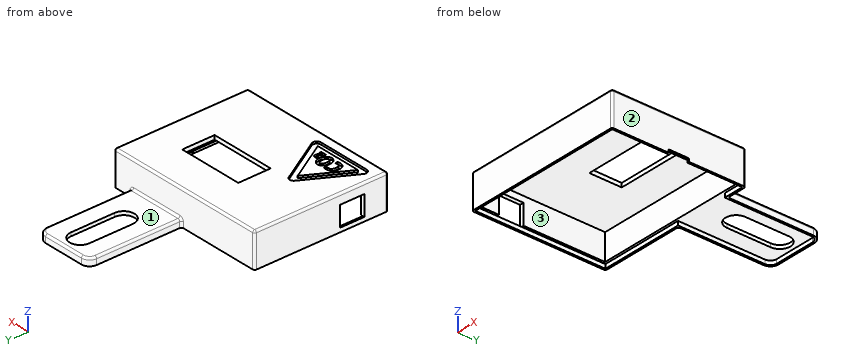
from build123d import *

# Parameters (mm, degrees)
CROQUIS1_W              = 80
CROQUIS1_H              = 66
SALIENTE_EXTRUIR2_DEPTH = 17
VACIADO7_T              = -2
CORTAR_EXTRUIR9_REACH   = 58.118
CROQUIS12_W             = 32
CROQUIS12_H             = 16
SALIENTE_EXTRUIR3_DEPTH = 3.75
CORTAR_EXTRUIR11_DEPTH  = 2
CORTAR_EXTRUIR26_REACH  = 117.461
CROQUIS16_W             = 10
CROQUIS16_H             = 12
CROQUIS20_RX            = 3.568577335
CROQUIS20_RY            = 2.914426882
CROQUIS20_RX_2          = 2.232634343
CROQUIS20_RY_2          = 1.215365865
CORTAR_EXTRUIR24_DEPTH  = 1
CORTAR_EXTRUIR25_REACH  = 117.461
CROQUIS27_W             = 1.5
CROQUIS27_H             = 10
REDONDEO3_R             = 1


with BuildPart() as part:
    # Croquis1 → Saliente-Extruir2 (new body)
    with BuildSketch(Plane.XY):
        with Locations((0, 2.5)):
            Rectangle(CROQUIS1_W, CROQUIS1_H)
    extrude(amount=SALIENTE_EXTRUIR2_DEPTH)

    # Vaciado7
    vaciado7_openings = [part.faces().sort_by_distance(p)[0] for p in [
        (0, 2.5, 0),
    ]]
    offset(amount=VACIADO7_T, openings=vaciado7_openings, kind=Kind.INTERSECTION)

    # Croquis12 → Cortar-Extruir9 (cut, up to next)
    with BuildSketch(Plane.XY.offset(17), mode=Mode.PRIVATE) as cortar_extruir9_sk1:
        with Locations((6.6, 9)):
            Rectangle(CROQUIS12_W, CROQUIS12_H)
    cortar_extruir9_tool1 = extrude(cortar_extruir9_sk1.sketch, amount=-CORTAR_EXTRUIR9_REACH, mode=Mode.PRIVATE) & part.part
    add(cortar_extruir9_tool1.solids().sort_by_distance((6.6, 9, 17))[0], mode=Mode.SUBTRACT)

    # Croquis29 → Saliente-Extruir3 (add)
    with BuildSketch(Plane(origin=(0, 0, 0), x_dir=(-1, 0, 0), z_dir=(0, 0, -1))):
        with BuildLine():
            Line((-1.5, 77.5), (-1.5, 35.5))
            Line((-1.5, 35.5), (-30, 35.5))
            Line((-30, 35.5), (-30, 77.5))
            ThreePointArc((-30, 77.5), (-28.828427125, 80.328427125), (-26, 81.5))
            Line((-26, 81.5), (-5.5, 81.5))
            ThreePointArc((-5.5, 81.5), (-2.671572875, 80.328427125), (-1.5, 77.5))
        make_face()
        with BuildLine():
            Line((-10.5, 73.25), (-10.5, 51.75))
            ThreePointArc((-10.5, 51.75), (-15.75, 46.5), (-21, 51.75))
            Line((-21, 51.75), (-21, 73.25))
            ThreePointArc((-21, 73.25), (-15.75, 78.5), (-10.5, 73.25))
        make_face(mode=Mode.SUBTRACT)
    extrude(amount=-SALIENTE_EXTRUIR3_DEPTH)

    # Croquis14 → Cortar-Extruir11 (cut)
    with BuildSketch(Plane(origin=(0, 0, 0), x_dir=(-1, 0, 0), z_dir=(0, 0, -1))):
        with BuildLine():
            Line((39.1, 34.6), (-2.4, 34.6))
            Line((-2.4, 34.6), (-2.4, 77.5))
            ThreePointArc((-2.4, 77.5), (-3.307968978, 79.692031022), (-5.5, 80.6))
            Line((-5.5, 80.6), (-26, 80.6))
            ThreePointArc((-26, 80.6), (-28.192031022, 79.692031022), (-29.1, 77.5))
            Line((-29.1, 77.5), (-29.1, 34.6))
            Line((-29.1, 34.6), (-39.1, 34.6))
            Line((-39.1, 34.6), (-39.1, -29.6))
            Line((-39.1, -29.6), (39.1, -29.6))
            Line((39.1, -29.6), (39.1, 34.6))
        make_face()
    extrude(amount=-CORTAR_EXTRUIR11_DEPTH, mode=Mode.SUBTRACT)

    # Croquis16 → Cortar-Extruir26 (cut, up to next)
    with BuildSketch(Plane.ZY.offset(40), mode=Mode.PRIVATE) as cortar_extruir26_sk1:
        with Locations((7, -12.75)):
            Rectangle(CROQUIS16_W, CROQUIS16_H)
    cortar_extruir26_tool1 = extrude(cortar_extruir26_sk1.sketch, amount=-CORTAR_EXTRUIR26_REACH, mode=Mode.PRIVATE) & part.part
    add(cortar_extruir26_tool1.solids().sort_by_distance((-40, -12.75, 7))[0], mode=Mode.SUBTRACT)

    # Croquis20 → Cortar-Extruir24 (cut)
    # profile 1 of 4: a face of its own
    with BuildSketch(Plane.XY.offset(17)):
        with BuildLine():
            Line((-18.590755698, -0.003579358), (-5.567484693, -22.587785135))
            ThreePointArc((-5.567484693, -22.587785135), (-5.568268134, -24.587332542), (-7.300057676, -25.586880154))
            Line((-7.300057676, -25.586880154), (-33.408883205, -25.586880154))
            ThreePointArc((-33.408883205, -25.586880154), (-35.141705867, -24.58554207), (-35.139387206, -22.584205777))
            Line((-35.139387206, -22.584205777), (-22.053832682, 0))
            ThreePointArc((-22.053832682, 0), (-20.321261528, 0.997324555), (-18.590755698, -0.003579358))
        make_face()
        Polygon((-8.62777783, -22.920674051), (-31.552205736, -22.920674051), (-20.06264827, -3.090980963), align=None, mode=Mode.SUBTRACT)
    # profile 2 of 4: a face of its own
    with BuildSketch(Plane.XY.offset(17)):
        with BuildLine():
            add(Edge.make_bspline(
                [(-22.220585459, -15.688668337), (-22.473316841, -15.63034571), (-22.720114648, -15.532860824), (-22.978779606, -15.513700456), (-23.250899762, -15.493543408), (-23.524824294, -15.535960138), (-23.795296381, -15.572023083), (-25.212214439, -15.760945491), (-25.122584621, -18.059259203), (-24.786781035, -18.954735434), (-24.397757557, -19.992131374), (-23.042460631, -19.849908777), (-22.220585459, -19.712929581)],
                knots=[0, 0, 0, 0, 1, 1, 1, 2, 2, 2, 3, 3, 3, 4, 4, 4, 4], degree=3))
            Line((-22.220585459, -19.712929581), (-22.103940205, -20.996027369))
            add(Edge.make_bspline(
                [(-22.103940205, -20.996027369), (-23.28060818, -21.143110866), (-24.188386831, -21.254263886), (-25.253362049, -20.762736862), (-25.303288102, -20.739694069), (-25.331125551, -20.68497336), (-25.370007302, -20.646091609), (-25.753754737, -20.262344174), (-26.08625723, -20.026013927), (-26.30316933, -19.537961701), (-27.149632898, -17.633418674), (-26.592646966, -15.27423428), (-24.611813155, -14.463893175), (-23.752583307, -14.112390056), (-22.840530525, -14.122598946), (-21.987294952, -14.463893175)],
                knots=[0, 0, 0, 0, 1, 1, 1, 2, 2, 2, 3, 3, 3, 4, 4, 4, 5, 5, 5, 5], degree=3))
            Line((-21.987294952, -14.463893175), (-22.220585459, -15.688668337))
        make_face()
    # profile 3 of 4: a face of its own
    with BuildSketch(Plane.XY.offset(17)):
        with Locations(Location((-18.587049995, -17.670107047), (0, 0, -90.640192277))):
            Ellipse(CROQUIS20_RX, CROQUIS20_RY)
        with Locations(Location((-18.601854743, -17.667818984), (0, 0, -89.299840613))):
            Ellipse(CROQUIS20_RX_2, CROQUIS20_RY_2, mode=Mode.SUBTRACT)
    # profile 4 of 4: a face of its own
    with BuildSketch(Plane.XY.offset(17)):
        with BuildLine():
            add(Edge.make_bspline(
                [(-15.455160758, -21.112672623), (-15.435719882, -20.85994124), (-15.496688009, -20.587461524), (-15.396838131, -20.354478475), (-15.283211235, -20.089349051), (-12.445503229, -17.671637646), (-14.463676103, -17.671637646), (-14.869932367, -17.671637646), (-14.884905464, -17.820686956), (-15.221870251, -17.904928152)],
                knots=[0, 0, 0, 0, 1, 1, 1, 2, 2, 2, 3, 3, 3, 3], degree=3))
            Line((-15.221870251, -17.904928152), (-15.455160758, -17.205056632))
            add(Edge.make_bspline(
                [(-15.455160758, -17.205056632), (-13.86644657, -16.410699538), (-12.632559042, -16.798398876), (-12.888965182, -18.721444927), (-12.955583326, -19.221081006), (-13.831530636, -19.988290714), (-14.113740343, -20.296155848)],
                knots=[0, 0, 0, 0, 1, 1, 1, 2, 2, 2, 2], degree=3))
            Line((-14.113740343, -20.296155848), (-12.712782774, -20.296155848))
            Line((-12.712782774, -20.296155848), (-12.712782774, -21.114840351))
            Line((-12.712782774, -21.114840351), (-15.455160758, -21.112672623))
        make_face()
    extrude(amount=-CORTAR_EXTRUIR24_DEPTH, mode=Mode.SUBTRACT)

    # Croquis27 → Cortar-Extruir25 (cut, up to next)
    with BuildSketch(Plane(origin=(40, 0, 0), x_dir=(0, 0, -1), z_dir=(1, 0, 0)), mode=Mode.PRIVATE) as cortar_extruir25_sk1:
        with Locations((-0.75, 2.5)):
            Rectangle(CROQUIS27_W, CROQUIS27_H)
    cortar_extruir25_tool1 = extrude(cortar_extruir25_sk1.sketch, amount=-CORTAR_EXTRUIR25_REACH, mode=Mode.PRIVATE) & part.part
    add(cortar_extruir25_tool1.solids().sort_by_distance((40, 2.5, 0.75))[0], mode=Mode.SUBTRACT)

    # Redondeo3
    redondeo3_edges = [part.edges().sort_by_distance(p)[0] for p in [
        (-40, 2.5, 17),
        (0, -30.5, 17),
        (28.828427125, 80.328427125, 3.75),
        (15.75, 81.5, 3.75),
        (2.671572875, 80.328427125, 3.75),
        (1.5, 56.5, 3.75),
        (15.75, 35.5, 3.75),
        (1.5, 35.5, 1.875),
        (30, 56.5, 3.75),
        (30, 35.5, 1.875),
        (40, 2.5, 17),
        (40, -30.5, 8.5),
        (-40, -30.5, 8.5),
        (-40, 35.5, 8.5),
        (40, 35.5, 8.5),
        (0, 35.5, 17),
    ]]
    fillet(redondeo3_edges, radius=REDONDEO3_R)


solid = part.part
Input: part model. Units: mm. Frame: model coordinates. Face numbers are marked on the shaded views. A direction names the side the tool comes from. Coordinates: 2 decimals unless noted, no trailing zeros. Order: outer loops, then holes, each group sorted by start corner. A loop starts at its lowest first (then second) coordinate and runs counter-clockwise, first axis right, second up.
1. Ray query, line 1 along Y through (x, z) = (0, 0.75); line 2 along X through (y, z) = (27, 5); line 3 along Y through (x, z) = (25, 12). Return the intervals inside material, ascending.
Checked values:
line 1: y = -30.5 to -29.6, 34.6 to 35.5
line 2: x = -40 to -38, 38 to 40
line 3: y = -30.5 to -28.5, 33.5 to 35.5
2. Cut plane C-C, the plane x = -2. Return loops of the section in (y, z).
Checked values:
outline: (-30.5, 0) - (-29.6, 0) - (-29.6, 2) - (-28.5, 2) - (-28.5, 15) - (1, 15) - (1, 17) - (-29.5, 17) arc R1 ccw to (-30.5, 16) - close; (17, 15) - (33.5, 15) - (33.5, 2) - (34.6, 2) - (34.6, 0) - (35.5, 0) - (35.5, 16) arc R1 ccw to (34.5, 17) - (17, 17) - close
3. Contact query for flat-ended pins moving along their axis: P1, Ø12, axis at x = 16.5, y = -9, coming from the -Z side; P2, Ø0.6, axis at y = 46.5, z = 1, coming from the +X side; P3, Ø0.6, axis at x = 1, z = 0.5, coming from the +Y side. Output: stop coordinate, or through.
Checked values:
P1: stops at z = 15
P2: stops at x = 30
P3: stops at y = 35.9
4. Cut plane A-A, the plane x = 15.75. Return loops of the section in (y, z).
Checked values:
outline: (-30.5, 0) - (-29.6, 0) - (-29.6, 2) - (-28.5, 2) - (-28.5, 15) - (1, 15) - (1, 17) - (-29.5, 17) arc R1 ccw to (-30.5, 16) - close; (17, 15) - (33.5, 15) - (33.5, 2) - (46.5, 2) - (46.5, 3.75) - (36.5, 3.75) arc R1 cw to (35.5, 4.75) - (35.5, 16) arc R1 ccw to (34.5, 17) - (17, 17) - close; (78.5, 2) - (80.6, 2) - (80.6, 0) - (81.5, 0) - (81.5, 2.75) arc R1 ccw to (80.5, 3.75) - (78.5, 3.75) - close
5. Cut plane D-D, the plane y = 24. Return loops of the section in (x, z), plus the area to 3 significant figures.
Checked values:
outline: (-40, 0) - (-39.1, 0) - (-39.1, 2) - (-38, 2) - (-38, 15) - (38, 15) - (38, 2) - (39.1, 2) - (39.1, 0) - (40, 0) - (40, 16) arc R1 ccw to (39, 17) - (-39, 17) arc R1 ccw to (-40, 16) - close
area: 215 mm2
6. Access query for the marked faces 1, 2 and 3. Directions: +Z, -Z, +X, -X, +Y, -Y. A direction counts if a zero-diameter tool reaches every point of the face in a straight line with its end or side. Return the directions, or none.
Checked values:
face 1: +Z, +X, -X, +Y
face 2: +Z, -Z, +X, +Y, -Y
face 3: -Z
7. Cut plane B-B, the plane z = 8.5. Return loops of the section in (x, y), plus the area to 3 significant figures.
Checked values:
outline: (-40, -29.5) arc R1 ccw to (-39, -30.5) - (39, -30.5) arc R1 ccw to (40, -29.5) - (40, 34.5) arc R1 ccw to (39, 35.5) - (-39, 35.5) arc R1 ccw to (-40, 34.5) - (-40, -6.75) - (-38, -6.75) - (-38, 33.5) - (38, 33.5) - (38, -28.5) - (-38, -28.5) - (-38, -18.75) - (-40, -18.75) - close
area: 543 mm2
